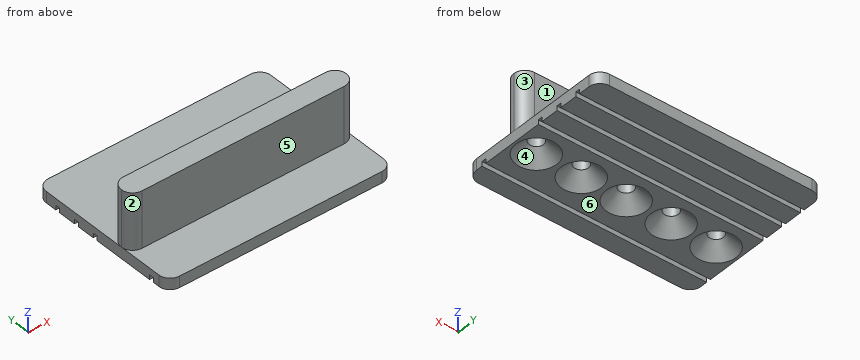
```python
from build123d import *

# Parameters (mm, degrees)
F0_W           = 50
F0_H           = 5
F0_H_2         = 4
F0_H_3         = 1
F1_DEPTH       = 2.5
F2_DEPTH       = 15
F3_R           = 2.49999
F4_D           = 3.2
F4_DEPTH       = 12
F4_CSINK_D     = 8.96
F4_CSINK_ANGLE = 90
F4_TIP         = 0.9613769904
F5_DEPTH       = 1


# Not quite as in the source:
# - a fillet or chamfer is up to 0.001 mm smaller than in the source, because OpenCascade refuses the exact size


with BuildPart() as f1:
    # F0 (on Top) → F1 (new body)
    with BuildSketch(Plane.XY):
        with Locations((0, 15)):
            Rectangle(F0_W, F0_H)
        with Locations((0, -5.5)):
            Rectangle(F0_W, F0_H_2)
        with Locations((0, -15.5)):
            Rectangle(F0_W, F0_H_2)
        with Locations((0, -13)):
            Rectangle(F0_W, F0_H_3)
        with Locations((0, -10.5)):
            Rectangle(F0_W, F0_H_2)
        with Locations((0, -3)):
            Rectangle(F0_W, F0_H_3)
        with Locations((0, -0.5)):
            Rectangle(F0_W, F0_H_2)
        with Locations((0, 7)):
            Rectangle(F0_W, F0_H_3)
        with Locations((0, 9.5)):
            Rectangle(F0_W, F0_H_2)
        with Locations((0, 12)):
            Rectangle(F0_W, F0_H_3)
        with Locations((0, -8)):
            Rectangle(F0_W, F0_H_3)
        with Locations((0, 2)):
            Rectangle(F0_W, F0_H_3)
        with Locations((0, 4.5)):
            Rectangle(F0_W, F0_H_2)
    extrude(amount=F1_DEPTH)

    # F0 (on Top) → F2 (join)
    with BuildSketch(Plane.XY):
        with Locations((0, -5.5)):
            Rectangle(F0_W, F0_H_2)
        with Locations((0, -3)):
            Rectangle(F0_W, F0_H_3)
    extrude(amount=F2_DEPTH)

    # F3 (radius 2.5 in the source; OpenCascade refuses exactly that, so slightly less here)
    f3_edges = [f1.edges().sort_by_distance(p)[0] for p in [
        (-25, 17.5, 1.25),
        (25, 17.5, 1.25),
        (25, -2.5, 8.75),
        (25, -7.5, 8.75),
        (-25, -2.5, 8.75),
        (-25, -7.5, 8.75),
        (-25, -17.5, 1.25),
        (25, -17.5, 1.25),
    ]]
    fillet(f3_edges, radius=F3_R)

    # F4
    with Locations(Plane(origin=(0, 0, 0), x_dir=(1, 0, 0), z_dir=(0, 0, -1))):
        with Locations((20, 5), (10, 5), (0, 5), (-10, 5), (-20, 5)):
            CounterSinkHole(F4_D / 2, F4_CSINK_D / 2, depth=F4_DEPTH, counter_sink_angle=F4_CSINK_ANGLE)
            with Locations((0, 0, -(F4_DEPTH + F4_TIP / 2))):  # 118° drill point
                Cone(0, F4_D / 2, F4_TIP, mode=Mode.SUBTRACT)

    # F0 (on Top) → F5 (cut)
    with BuildSketch(Plane.XY):
        with Locations((0, -13)):
            Rectangle(F0_W, F0_H_3)
        with Locations((0, 2)):
            Rectangle(F0_W, F0_H_3)
        with Locations((0, 7)):
            Rectangle(F0_W, F0_H_3)
        with Locations((0, 12)):
            Rectangle(F0_W, F0_H_3)
    extrude(amount=F5_DEPTH, mode=Mode.SUBTRACT)


solid = f1.part
```
Build history of the part. All positions in model axes, mm. Face numbers are marked on the shaded views. A direction names the side the tool comes from. Round coordinates to 2 decimals unless told otherwise and drop trailing zeros. Write each loop counter-clockwise with the first axis right and the second up, starting at its lowest first coordinate (ties: lowest second). Pieces come first, ordered by that corner, then holes.
1) 3-axis set-ups, long thin cutter, end or side, ignore diameter. For the marked faces 1, 2 and 3: which of +Z, -Z, +X, -X, +Y, -Y reach the whole face in a straight line?
2) Mould opens along Y. For the marked faces 4, 5 and 6 say: +Y half, -Y half, draft (parallel to the pull), parting line (faces both ways), or undercut.
3) Pin check, flat tips, straight feed: pin 1 (3.5 mm diameter, centred on x = 0, y = -5, fed in from -Z); pin 2 (0.8 mm diameter, centred on x = -1, y = -13, fed in from -Z); pin 3 (4 mm diameter, centred on x = 12.5, z = 9.5, fed in from +Y). Stop position of each tip, or through.
4) Band-saw the part on B-B, the plane y = 5. List the corners of the cut face in (x, z).
5) Drill centre lines: probe 1 along X at (y, z) = (-5, 5); probe 2 along Y at (x, z) = (0, 10.25); probe 3 along Z at (x, y) = (9, 11). Where is each one in solid material? Low to high.
Ans:
1. face 1: +Z, +X, -X, +Y
1. face 2: +Z, -X, -Y
1. face 3: +Z, +X, +Y
2. face 4: undercut
2. face 5: -Y half
2. face 6: draft
3. pin 1: stops at z = 2.73
3. pin 2: stops at z = 1
3. pin 3: stops at y = -2.5
4. outline: (-25, 0) - (25, 0) - (25, 2.5) - (-25, 2.5) - close
5. probe 1: x = -25 to -21.6, -18.4 to -11.6, -8.4 to -1.6, 1.6 to 8.4, 11.6 to 18.4, 21.6 to 25
5. probe 2: y = -7.5 to -6.6, -3.4 to -2.5
5. probe 3: z = 0 to 2.5
